Check sheet for the modelled part. Datum: model origin and axes. Units: mm. Give positions to 0.01 mm unless a question says otherwise; leave off trailing zeros. Write each loop counter-clockwise with the first axis right and the second up, starting at its lowest first coordinate (ties: lowest second). Pieces come first, ordered by that corner, then holes. Notation, with made-up numbers: (10.5, 62.25) -> (37.5, 62.25) arc R30 ccw to (37.5, 84.25) -> close; hole circle Ø7 at (85, 0). An arc over 180 degrees is marked (long way). Use a Markdown table: item, result. Add a question column.
1. Scan lines: probe 1 along X at (y, z) = (3.75, 1); probe 2 along Z at (x, y) = (759, -4.5); probe 3 along X at (y, z) = (-5, -3.25). Record each from-to range of solid material in increasing order. Write a range as [from, to].
2. Cross-section at A-A (x = 193.5). Enter the section's corners in (y, z), then the cut area to 3 significant figures.
3. Gauge pin test, flat ends, axial feed: P1, Ø2, axis at x = 742, z = 4.5, coming from the -Y side; P2, Ø4, axis at y = -4, z = -4, coming from the +X side; P3, Ø6, axis at x = 762, z = -3.5, coming from the -Y side. Record the tip position at first contact, or that the pin passes through.
Autodesk Inventor part; units mm, degrees
ref_plane "YZ Plane" through (0, 0, 0) normal (1, 0, 0) x (0, 1, 0)
ref_plane "XZ Plane" through (0, 0, 0) normal (0, 1, 0) x (-1, 0, 0)
ref_plane "XY Plane" through (0, 0, 0) normal (0, 0, 1) x (1, 0, 0)
sketch "Sketch1" plane through (0, 0, 0) normal (0, 0, 1) x (1, 0, 0)
  line L0 (0, 4) -> (1, 4) construction
  line L1 (15, 4) -> (16, 5)
  line L2 (16, 5) -> (54, 5)
  line L3 (0, 4) -> (0, 3) construction
  line L4 (54, 5) -> (55, 6)
  line L5 (55, 6) -> (1089, 6)
  line L6 (0, 3) -> (1, 4)
  line L7 (0, 3) -> (0, 0)
  line L8 (1, 4) -> (15, 4)
  line L9 (1089, 6) -> (1090, 5)
  line L10 (1090, 5) -> (1090, 4)
  line L11 (1090, 4) -> (1097, 4)
  line L12 (1097, 4) -> (1097, 3.8)
  line L13 (1097, 3.8) -> (1097.9, 3.8)
  line L14 (1097.9, 3.8) -> (1097.9, 4)
  line L15 (1097.9, 4) -> (1099, 4)
  line L16 (1099, 4) -> (1100, 3)
  line L17 (1100, 3) -> (1100, 0)
  line L18 (0, 0) -> (1100, 0)
  point P0 (0, 0)
  point P1 (1100, 1.5)
  dimension "d0" = 4
  dimension "d1" = 5
  dimension "d2" = 6
  dimension "d3" = 135
  dimension "d4" = 135
  dimension "d5" = 15
  dimension "d6" = 39
  dimension "d7" = 135
  dimension "d8" = 4
  dimension "d9" = 7
  dimension "d10" = 10
  dimension "d11" = 0.2
  dimension "d12" = 0.9
  dimension "d14" = 135
  dimension "d15" = 1100
revolve "Revolution1" add sketch "Sketch1" angle 360 about axis through (0, 0, 0) along (1, 0, 0)
equation "\"SHAFT_LEN\" = 1100"
properties part number "SFU1204-800"
Worked answers:
| question | item | result |
|---|---|---|
| 1 | probe 1 | x = [0.88, 1097], [1097.9, 1099.12] |
| 1 | probe 2 | z = [-3.97, 3.97] |
| 1 | probe 3 | x = [54.96, 1089.04] |
| 2 | outline | circle Ø12 at (0, 0) |
| 2 | area | 113 mm² |
| 3 | P1 | stops at y = -4.87 |
| 3 | P2 | stops at x = 1099.34 |
| 3 | P3 | stops at y = -5.98 |
